Design review of the part built by this model. Coordinates are the model's own, in mm. A direction names the side the tool comes from. Give positions to 0.01 mm unless a question says otherwise; leave off trailing zeros. Loops run counter-clockwise (first coordinate to the right, second up) from the corner with the lowest first, then second, coordinate; pieces in that order, holes last. Notation, with made-up numbers: (31, 71) -> (58, 71) arc R18 cw to (58, 79) -> close; hole circle Ø8 at (13, 20.25). An arc over 180 degrees is marked (long way). Answer as CSV lines item,"result".
Autodesk Inventor part; units mm, degrees
ref_plane "YZ Plane" through (0, 0, 0) normal (1, 0, 0) x (0, 1, 0)
ref_plane "XZ Plane" through (0, 0, 0) normal (0, 1, 0) x (-1, 0, 0)
ref_plane "XY Plane" through (0, 0, 0) normal (0, 0, 1) x (1, 0, 0)
sketch "Sketch2" plane through (0, 0, 0) normal (0, 0, 1) x (1, 0, 0)
  circle A0 centre (0, 0) radius 1.5
  dimension "Diameter" = 3
extrude "Extrusion1" add sketch "Sketch2" against normal blind 8.14
sketch "Sketch3" plane through (0, 0, 0) normal (0, 0, 1) x (1, 0, 0)
  circle A0 centre (0, 0) radius 1.5
extrude "Extrusion2" add sketch "Sketch3" along normal blind 1.86 draft 45
sketch "Sketch4" plane through (0, 0, 1.86) normal (0, 0, 1) x (1, 0, 0)
  circle A0 centre (0, 0) radius 3.36
  line L0 (0.5774, 1) -> (1.1547, 0)
  line L1 (1.1547, 0) -> (0.5774, -1)
  line L2 (0.5774, -1) -> (-0.5774, -1)
  line L3 (-0.5774, -1) -> (-1.1547, 0)
  line L4 (-1.1547, 0) -> (-0.5774, 1)
  line L5 (-0.5774, 1) -> (0.5774, 1)
  line L6 (0, 0) -> (1.1547, 0) construction
  dimension "Hex_Width" = 2
extrude "Extrusion3" cut sketch "Sketch4" against normal blind 1.1 contours L0 L1 L2 L3 L4 L5
thread "Thread1"
chamfer "Chamfer1" distance 0.3 angle 45 1 edges at (-1.5, 0, -8.14)
fillet "Fillet1" radius 0.1 1 edges at (-3.36, 0, 1.86)
equation "\"Length1\" = Length - Head_Height"
equation "\"Thread_Length\" = Length1"
equation "\"Length\" = 10"
properties part number "SCREW,FLAT-HD,P,10_9,M03X0_50X010MM" material "Steel, MS"
Q1. We need section C-C, the plane z = -6.25. State the section outline as (x, y) points, and give its area (3 significant figures).
Filled sheet:
outline,"circle Ø3 at (0, 0)"
area,"7.07 mm^2"
Q2. For faces 5 (the flat face through (0.86, 0.51, 1.32)), 6 (the conical face through (-0.35, -1.57, 0.11)), list the 3-axis set-ups (+Z, -Z, +X, -X, +Y, -Y) from which the entire face can be reached by the end or side of a thin tool; tool diameter is ignored.
Filled sheet:
face 5,"+Z"
face 6,"-Z"
Q3. We need section B-B, the plane z = 0.5. State the section outline as (x, y) points.
Filled sheet:
outline,"circle Ø4 at (0, 0)"
Q4. The part is to be moulded in two halves that separate along Y. For faces 1 (the flat face through (0, 0, 0.76)), 2 (the flat face through (0, 0, -8.14)), 3 (the cylindrical face through (-1.5, 0.07, -3.87)), 4 (the flat face through (-0.87, 0.49, 1.32)), say which applies: pulls with the +Y half, pulls with the -Y half, needs draft (parallel to the pull), parting line crosses it, or undercut.
Filled sheet:
face 1,"undercut"
face 2,"needs draft"
face 3,"parting line crosses it"
face 4,"undercut"
Q5. To check wall thickness, follow probe 1 along X at (y, z) = (0, -6); probe 2 along Z at (x, y) = (0.75, -0.5); probe 3 along Z at (x, y) = (-0.5, -3). State the ranges of each line that lie inside material, in increasing order. Write a range as from..to.
Filled sheet:
probe 1,"x = -1.5..1.5"
probe 2,"z = -8.14..0.76"
probe 3,"z = 1.54..1.86"
Q6. Clearance check with flat-ended pins moving along their axes: pin 1 Ø2 at (y, z) = (-2, -2.5) entering from -X; pin 2 Ø2 at (x, z) = (-2, -4.5) entering from -Y. State where each tip first meets the part, or that it passes through.
Filled sheet:
pin 1,"stops at x = -1.12"
pin 2,"stops at y = -1.12"
Q7. We need section A-A, the plane x = 0. State the section outline as (y, z) points, and give its area (3 significant figures).
Filled sheet:
outline,"(-3.19, 1.69) -> (-1.5, 0) -> (-1.5, -7.84) -> (-1.2, -8.14) -> (1.2, -8.14) -> (1.5, -7.84) -> (1.5, 0) -> (3.19, 1.69) arc R0.1 ccw to (3.12, 1.86) -> (1, 1.86) -> (1, 0.76) -> (-1, 0.76) -> (-1, 1.86) -> (-3.12, 1.86) arc R0.1 ccw to start"
area,"31.1 mm^2"
